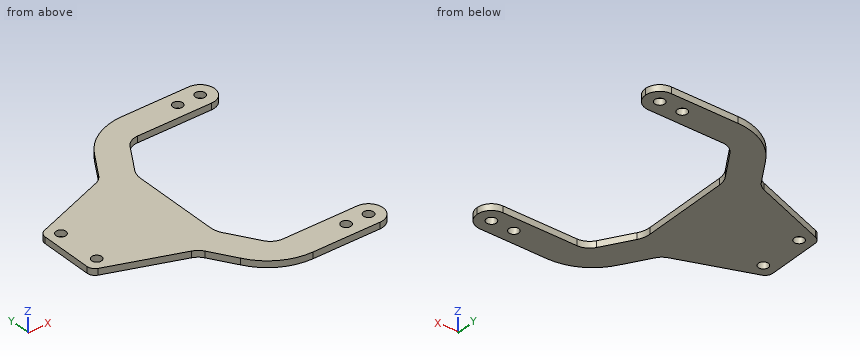
from build123d import *

# Parameters (mm, degrees)
F0_R     = 1.55
F1_DEPTH = 2


# Not quite as in the source:
# - a feature names something its author has since deleted; it is built from what else it names


with BuildPart() as f1:
    # F0 (on Top) → F1 (new body)
    with BuildSketch(Plane.XY):
        with BuildLine():
            Line((25.4436091884, 28.55), (48.5000015985, 28.55))
            ThreePointArc((48.5000015985, 28.55), (51.6819821139, 29.8680194847), (53.0000015985, 33.05))
            ThreePointArc((53.0000015985, 33.05), (51.6819821139, 36.2319805153), (48.5000015985, 37.55))
            Line((48.5000015985, 37.55), (27.6442359668, 37.55))
            ThreePointArc((27.6442359668, 37.55), (18.7122132684, 35.1775068554), (12.1347641944, 28.6854411684))
            Line((12.1347641944, 28.6854411684), (7.2011388972, 20.8408842798))
            ThreePointArc((7.2011388972, 20.8408842798), (6.1134719977, 19.6156574256), (4.6881494145, 18.8077863577))
            Line((4.6881494145, 18.8077863577), (-17.8597609739, 10.5497599571))
            ThreePointArc((-17.8597609739, 10.5497599571), (-19.0493172564, 9.6341347233), (-19.5, 8.2022482814))
            Line((-19.5, 8.2022482814), (-19.5, -8.2022482814))
            ThreePointArc((-19.5, -8.2022482814), (-19.0493172564, -9.6341347233), (-17.8597609739, -10.5497599571))
            Line((-17.8597609739, -10.5497599571), (4.6881494145, -18.8077863577))
            ThreePointArc((4.6881494145, -18.8077863577), (6.1134719977, -19.6156574256), (7.2011388972, -20.8408842798))
            Line((7.2011388972, -20.8408842798), (12.1347641944, -28.6854411684))
            ThreePointArc((12.1347641944, -28.6854411684), (18.7122132684, -35.1775068554), (27.6442359668, -37.55))
            Line((27.6442359668, -37.55), (48.5000015985, -37.55))
            ThreePointArc((48.5000015985, -37.55), (51.6819821139, -36.2319805153), (53.0000015985, -33.05))
            ThreePointArc((53.0000015985, -33.05), (51.6819821139, -29.8680194847), (48.5000015985, -28.55))
            Line((48.5000015985, -28.55), (25.4436091884, -28.55))
            ThreePointArc((25.4436091884, -28.55), (23.0259271525, -27.9266212509), (21.211097758, -26.2119254294))
            Line((21.211097758, -26.2119254294), (15.6422879472, -17.3574132338))
            ThreePointArc((15.6422879472, -17.3574132338), (14.8417868513, -15.5699685166), (14.5678039498, -13.6307176327))
            Line((14.5678039498, -13.6307176327), (14.5678039498, 13.6307176327))
            ThreePointArc((14.5678039498, 13.6307176327), (14.8417868513, 15.5699685166), (15.6422879472, 17.3574132338))
            Line((15.6422879472, 17.3574132338), (21.211097758, 26.2119254294))
            ThreePointArc((21.211097758, 26.2119254294), (23.0259271525, 27.9266212509), (25.4436091884, 28.55))
        make_face()
        with Locations((-15.55, -7)):
            Circle(F0_R, mode=Mode.SUBTRACT)
        with Locations((41.5000015985, -33.05)):
            Circle(F0_R, mode=Mode.SUBTRACT)
        with Locations((48.5000015985, -33.05)):
            Circle(F0_R, mode=Mode.SUBTRACT)
        with Locations((-15.55, 7)):
            Circle(F0_R, mode=Mode.SUBTRACT)
        with Locations((41.5000015985, 33.05)):
            Circle(F0_R, mode=Mode.SUBTRACT)
        with Locations((48.5000015985, 33.05)):
            Circle(F0_R, mode=Mode.SUBTRACT)
    extrude(amount=F1_DEPTH)


solid = f1.part
Work out the finished part from the listing and answer in its coordinate system (mm). Give positions to 0.01 mm unless a question says otherwise; leave off trailing zeros. Order: outer loops, then holes, each group sorted by start corner. A loop starts at its lowest first (then second) coordinate and runs counter-clockwise, first axis right, second up. Notation, with made-up numbers: M 76,-32.5 L 112,-32.5 A14 ccw 112,-10.5 Z; hole C 7.5,79.5 d4. An arc over 180 degrees is marked long. Return JSON: item names as keys, results as strings.
Q1. This flat-tipped pin is pushed along its axis until it touches: pin 1 (1 mm diameter, centred on y = 27.5, z = 0.5, fed in from -X). Where does it stop, or does it pass through?
Answer below:
{"pin 1": "stops at x = 11.07"}
Q2. Find section D-D, the plane x = -15.55. Write down the section's boundary in (y, z), and give its area (3 significant figures).
Answer below:
{"outline": "M -11.4,0 L -8.55,0 L -8.55,2 L -11.4,2 Z; M -5.45,0 L 5.45,0 L 5.45,2 L -5.45,2 Z; M 8.55,0 L 11.4,0 L 11.4,2 L 8.55,2 Z", "area": "33.2 mm^2"}
Q3. Find section B-B, the plane y = 7. Write down the section's boundary in (x, z), and give its area (3 significant figures).
Answer below:
{"outline": "M -19.5,0 L -17.1,0 L -17.1,2 L -19.5,2 Z; M -14,0 L 14.57,0 L 14.57,2 L -14,2 Z", "area": "61.9 mm^2"}
Q4. Find the intervals of material crossed by line 1 along Y through (x, z) = (27.5, 0.9); line 2 along Y through (x, z) = (-15.55, 0.65), in increasing order. Write a range as [from, to].
Answer below:
{"line 1": "y = [-37.55, -28.55], [28.55, 37.55]", "line 2": "y = [-11.4, -8.55], [-5.45, 5.45], [8.55, 11.4]"}
Q5. Find section C-C, the plane z = 0.55. State how many separate pieces and enclosed holes the cut face has, and give its area (3 significant figures).
Answer below:
{"separate pieces": "1", "enclosed holes": "6", "area": "1,880 mm^2"}
Q6. Find section A-A, the plane x = 30.5. Write down the section's boundary in (y, z).
Answer below:
{"outline": "M -37.55,0 L -28.55,0 L -28.55,2 L -37.55,2 Z; M 28.55,0 L 37.55,0 L 37.55,2 L 28.55,2 Z"}
